Could you check a few things on this model? Use its own coordinates, in mm. Face numbers are marked on the shaded views. A direction names the side the tool comes from. Round coordinates to 2 decimals unless told otherwise and drop trailing zeros. Loops run counter-clockwise (first coordinate to the right, second up) from the corner with the lowest first, then second, coordinate; pieces in that order, holes last. Notation, with made-up numbers: (80, 38) -> (96, 38) arc R25 ccw to (96, 71) -> close; hole circle Ø10 at (65.25, -33.75). An arc over 180 degrees is marked (long way). Write each question's results on one line, items separated by ' | '. Start each with the question number.
1) Imagine slicing it at B-B, the plane z = 0. List the corners of the cut face in (x, y) for me.
2) For P1, Ø8, axis at x = -25.5, y = 57.5, coming from the +Z side; P2, Ø20, axis at x = -0.5, y = 34.5, coming from the -Z side; P3, Ø7, axis at x = -30, z = 30, coming from the +Y side; P4, Ø1, axis at x = 20, y = 46, coming from the +Z side, each with a flat end and sliding along its axis, tell me the tip position at first contact or that it passes through.
3) Imagine slicing it at C-C, the plane y = 25. List the corners of the cut face in (x, z) for me, plus the area to 3 significant figures.
4) Imagine slicing it at A-A, the plane x = 0. List the corners of the cut face in (y, z) for me.
5) Which directions (+Z, -Z, +X, -X, +Y, -Y) give clear straight access to the entire face, cutting with the end or side of a thin tool? Please do the marked faces 1, 2, 3, 4 and 5.
6) Imagine slicing it at D-D, the plane z = -8. List the corners of the cut face in (x, y) for me, plus the area to 3 significant figures.
7) If I drill on probe 1 along Z at (x, y) = (-30, 52.8); probe 2 along X at (y, z) = (53.85, 0), over which ranges is the centre line in solid material (lowest first)?
from build123d import *

# Parameters (mm, degrees)
SKETCH1_W           = 50
SKETCH1_H           = 50
BOSS_EXTRUDE1_DEPTH = 50
SKETCH2_W           = 70
SKETCH2_H           = 70
SKETCH2_R           = 3
BOSS_EXTRUDE2_DEPTH = 5
FILLET1_R           = 5
FILLET2_R           = 5
SKETCH3_R           = 19.851731711
SKETCH3_R_2         = 16.528882373
CUT_EXTRUDE1_DEPTH  = 3
SKETCH4_R           = 5
BOSS_EXTRUDE3_DEPTH = 20


with BuildPart() as part:
    # Sketch1 → Boss-Extrude1 (new body)
    with BuildSketch(Plane(origin=(0, 0, 0), x_dir=(1, 0, 0), z_dir=(0, 1, 0))):
        Rectangle(SKETCH1_W, SKETCH1_H)
    extrude(amount=BOSS_EXTRUDE1_DEPTH)

    # Sketch2 → Boss-Extrude2 (add)
    with BuildSketch(Plane(origin=(0, 50, 0), x_dir=(1, 0, 0), z_dir=(0, 1, 0))):
        Rectangle(SKETCH2_W, SKETCH2_H)
        with Locations((-30, 30)):
            Circle(SKETCH2_R, mode=Mode.SUBTRACT)
        with Locations((30, 30)):
            Circle(SKETCH2_R, mode=Mode.SUBTRACT)
        with Locations((-30, -30)):
            Circle(SKETCH2_R, mode=Mode.SUBTRACT)
        with Locations((30, -30)):
            Circle(SKETCH2_R, mode=Mode.SUBTRACT)
    extrude(amount=BOSS_EXTRUDE2_DEPTH)

    # Fillet1
    fillet1_edges = [part.edges().sort_by_distance(p)[0] for p in [
        (25, 25, 25),
        (-25, 25, 25),
        (-25, 25, -25),
        (25, 25, -25),
    ]]
    fillet(fillet1_edges, radius=FILLET1_R)

    # Fillet2
    fillet2_edges = [part.edges().sort_by_distance(p)[0] for p in [
        (35, 52.5, 35),
        (35, 52.5, -35),
        (-35, 52.5, -35),
        (-35, 52.5, 35),
    ]]
    fillet(fillet2_edges, radius=FILLET2_R)

    # Sketch3 → Cut-Extrude1 (cut)
    with BuildSketch(Plane(origin=(0, 55, 0), x_dir=(1, 0, 0), z_dir=(0, 1, 0))):
        Circle(SKETCH3_R)
        Circle(SKETCH3_R_2, mode=Mode.SUBTRACT)
    extrude(amount=-CUT_EXTRUDE1_DEPTH, mode=Mode.SUBTRACT)

    # Sketch4 → Boss-Extrude3 (add)
    with BuildSketch(Plane(origin=(0, 55, 0), x_dir=(1, 0, 0), z_dir=(0, 1, 0))):
        Circle(SKETCH4_R)
    extrude(amount=BOSS_EXTRUDE3_DEPTH)


solid = part.part
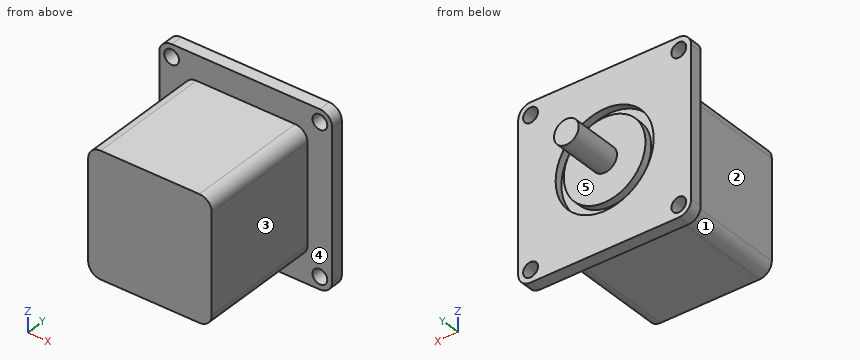
Checked values:
1) outline: (-35, 50) -> (-25, 50) -> (-25, 0) -> (25, 0) -> (25, 50) -> (35, 50) -> (35, 55) -> (19.85, 55) -> (19.85, 52) -> (16.53, 52) -> (16.53, 55) -> (5, 55) -> (5, 75) -> (-5, 75) -> (-5, 55) -> (-16.53, 55) -> (-16.53, 52) -> (-19.85, 52) -> (-19.85, 55) -> (-35, 55) -> close
2) P1: z = 35 | P2: z = -25 | P3: y = 55 | P4: z = 25
3) outline: (-25, -20) arc R5 ccw to (-20, -25) -> (20, -25) arc R5 ccw to (25, -20) -> (25, 20) arc R5 ccw to (20, 25) -> (-20, 25) arc R5 ccw to (-25, 20) -> close | area: 2,480 mm^2
4) outline: (0, -25) -> (50, -25) -> (50, -35) -> (55, -35) -> (55, -19.85) -> (52, -19.85) -> (52, -16.53) -> (55, -16.53) -> (55, -5) -> (75, -5) -> (75, 5) -> (55, 5) -> (55, 16.53) -> (52, 16.53) -> (52, 19.85) -> (55, 19.85) -> (55, 35) -> (50, 35) -> (50, 25) -> (0, 25) -> close
5) face 1: -Z, -X, -Y | face 2: +Z, -Z, -X, -Y | face 3: +Z, -Z, +X, -Y | face 4: -Y | face 5: +Y
6) outline: (-35, 50) -> (-25, 50) -> (-25, 0) -> (25, 0) -> (25, 50) -> (35, 50) -> (35, 55) -> (18.17, 55) -> (18.17, 52) -> (14.46, 52) -> (14.46, 55) -> (-14.46, 55) -> (-14.46, 52) -> (-18.17, 52) -> (-18.17, 55) -> (-35, 55) -> close | area: 2,830 mm^2
7) probe 1: -35 to -33, -27 to 27, 33 to 35 | probe 2: -35 to -19.85, -16.53 to 16.53, 19.85 to 35
